Autodesk Inventor part; units mm, degrees
ref_plane "YZ Plane" through (0, 0, 0) normal (1, 0, 0) x (0, 1, 0)
ref_plane "XZ Plane" through (0, 0, 0) normal (0, 1, 0) x (-1, 0, 0)
ref_plane "XY Plane" through (0, 0, 0) normal (0, 0, 1) x (1, 0, 0)
sketch "Sketch Base" plane through (0, 0, 0) normal (0, 0, 1) x (1, 0, 0)
  line L0 (0, 0) -> (36, 0)
  line L1 (36, 0) -> (36, 36)
  line L2 (36, 36) -> (0, 36)
  line L3 (0, 36) -> (0, 0)
  line L4 (0, 0) -> (36, 36) construction
  line L5 (36, 0) -> (0, 36) construction
  line L6 (3, 3) -> (33, 3) construction
  line L7 (33, 3) -> (33, 33) construction
  line L8 (33, 33) -> (3, 33) construction
  line L9 (3, 33) -> (3, 3) construction
  line L10 (3, 3) -> (33, 33) construction
  line L11 (33, 3) -> (3, 33) construction
  circle A0 centre (3, 33) radius 1.5
  circle A1 centre (33, 3) radius 1.5
  circle A2 centre (3, 33) radius 2.5
  circle A3 centre (33, 3) radius 2.5
  line L12 (-1, -1) -> (37, -1)
  line L13 (37, -1) -> (37, 37)
  line L14 (37, 37) -> (-1, 37)
  line L15 (-1, 37) -> (-1, -1)
  line L16 (-1, -1) -> (37, 37) construction
  line L17 (37, -1) -> (-1, 37) construction
  line L18 (-3, -3) -> (39, -3)
  line L19 (39, -3) -> (39, 39)
  line L20 (39, 39) -> (-3, 39)
  line L21 (-3, 39) -> (-3, -3)
  line L22 (-3, -3) -> (39, 39) construction
  line L23 (39, -3) -> (-3, 39) construction
  point P0 (18, 18)
  dimension "d0" = 36
  dimension "d1" = 36
  dimension "d2" = 30
  dimension "d3" = 30
  dimension "d4" = 3
  dimension "d6" = 3
  dimension "d8" = 5
  dimension "d11" = 5
  dimension "d12" = 38
  dimension "d13" = 38
  dimension "d14" = 42
  dimension "d15" = 42
extrude "Extrusion1" add sketch "Sketch Base" against normal blind 5 contours A2 | A3
extrude "Extrusion5" add sketch "Sketch Base" along normal blind 2 contours L3 L2 L1 L0 | A0 | A1 | A2 | A3 | L15 L14 L13 L12 | L21 L20 L19 L18
sketch "Sketch2" plane through (0, 0, 2) normal (0, 0, 1) x (1, 0, 0)
  line L0 (-3, 39) -> (-3, -3)
  line L1 (39, -3) -> (39, 39)
  line L2 (-3, -3) -> (39, -3)
  line L3 (39, -3) -> (39, 39)
  line L4 (39, 39) -> (-3, 39)
  line L5 (-3, 39) -> (-3, -3)
  line L6 (-3, -3) -> (39, 39) construction
  line L7 (-1.2, -1.2) -> (37.2, -1.2)
  line L8 (37.2, -1.2) -> (37.2, 37.2)
  line L9 (37.2, 37.2) -> (-1.2, 37.2)
  line L10 (-1.2, 37.2) -> (-1.2, -1.2)
  line L11 (-1.2, -1.2) -> (37.2, 37.2) construction
  line L12 (37.2, -1.2) -> (-1.2, 37.2) construction
  point P0 (0, 0)
  point P1 (18, 18)
  dimension "d30" = 38.4
  dimension "d31" = 38.4
extrude "Extrusion8" add sketch "Sketch2" along normal blind 1
fillet "Fillet1" radius 2 8 edges at (-3, -3, 1.5) (-3, 39, 1.5) (39, 39, 1.5) (39, -3, 1.5) (-1.2, 37.2, 2.5) (37.2, 37.2, 2.5) (37.2, -1.2, 2.5) (-1.2, -1.2, 2.5)
fillet "Fillet2" radius 2 2 edges at (0.5, 33, 0) (30.5, 3, 0)
properties part number "Controller Mount"
Build history of the part. All positions in model axes, mm. A direction names the side the tool comes from. Coordinates: 2 decimals unless noted, no trailing zeros. Order: outer loops, then holes, each group sorted by start corner. A loop starts at its lowest first (then second) coordinate and runs counter-clockwise, first axis right, second up.
Item 1: Saw through at C-C on x = 3. List the corners of the cut face in (y, z).
Filled in:
outline: (-3, 0) - (28.5, 0) arc R2 cw to (30.5, -2) - (30.5, -5) - (31.5, -5) - (31.5, 0) - (34.5, 0) - (34.5, -5) - (35.5, -5) - (35.5, -2) arc R2 cw to (37.5, 0) - (39, 0) - (39, 3) - (37.2, 3) - (37.2, 2) - (-1.2, 2) - (-1.2, 3) - (-3, 3) - close
Item 2: Mould opens along Y. For faces 1 (the cylindrical face through (4.34, 35.11, -3.48)), 2 (the flat face through (18, 39, 1)), 3 (the flat face through (18.2, 37.2, 2.5)) say: released by +Y, released by -Y, zero draft, split by the parting line, or undercut.
Filled in:
face 1: split by the parting line
face 2: released by +Y
face 3: undercut
Item 3: Saw through at D-D on y = 15.5. List the corners of the cut face in (x, z).
Filled in:
outline: (-3, 0) - (39, 0) - (39, 3) - (37.2, 3) - (37.2, 2) - (-1.2, 2) - (-1.2, 3) - (-3, 3) - close
Item 4: Saw through at A-A on z = -4.25. List the corners of the cut face in (x, y), then the cut area to 3 significant figures.
Filled in:
outline: circle Ø5 at (3, 33); circle Ø5 at (33, 3); hole circle Ø3 at (3, 33); hole circle Ø3 at (33, 3)
area: 25.1 mm2
Item 5: Tool access for faces 4 (the flat face through (18, 18, 2)), 5 (the flat face through (33, 3, 0)), 6 (the flat face through (-2, 18, 3)): list every direction of +Z, -Z, +X, -X, +Y, -Y with a clear straight run to the whole face (end or side of a thin tool).
Filled in:
face 4: +Z
face 5: -Z
face 6: +Z, +X, -X, +Y, -Y
Item 6: Saw through at B-B on y = 33. List the corners of the cut face in (x, z), then the cut area to 3 significant figures.
Filled in:
outline: (-3, 0) - (-1.5, 0) arc R2 cw to (0.5, -2) - (0.5, -5) - (1.5, -5) - (1.5, 0) - (4.5, 0) - (4.5, -5) - (5.5, -5) - (5.5, -2) arc R2 cw to (7.5, 0) - (39, 0) - (39, 3) - (37.2, 3) - (37.2, 2) - (-1.2, 2) - (-1.2, 3) - (-3, 3) - close
area: 99.3 mm2
Item 7: Drop flat-ended pins along their axis: pin 1 Ø10 at (x, y) = (6, 34.5) entering from -Z; pin 2 Ø3.5 at (x, y) = (3, 33) entering from +Z; pin 3 Ø4 at (x, y) = (6.5, 28.5) entering from -Z; pin 4 Ø12.5 at (x, y) = (15, 20.5) entering from -Z. Give the stop position or say it passes through.
Filled in:
pin 1: stops at z = -5
pin 2: stops at z = 2
pin 3: stops at z = -0.17
pin 4: stops at z = 0
Item 8: Drill centre lines: L1, parallel to Y at x = 3, z = -2.5; L2, parallel to Z at x = 36, y = 29; L3, parallel to X at y = 32, z = -1.5. Where is each one in solid material? Low to high.
Filled in:
L1: y = 30.5 to 31.5, 34.5 to 35.5
L2: z = 0 to 2
L3: x = 0.64 to 1.88, 4.12 to 5.36
